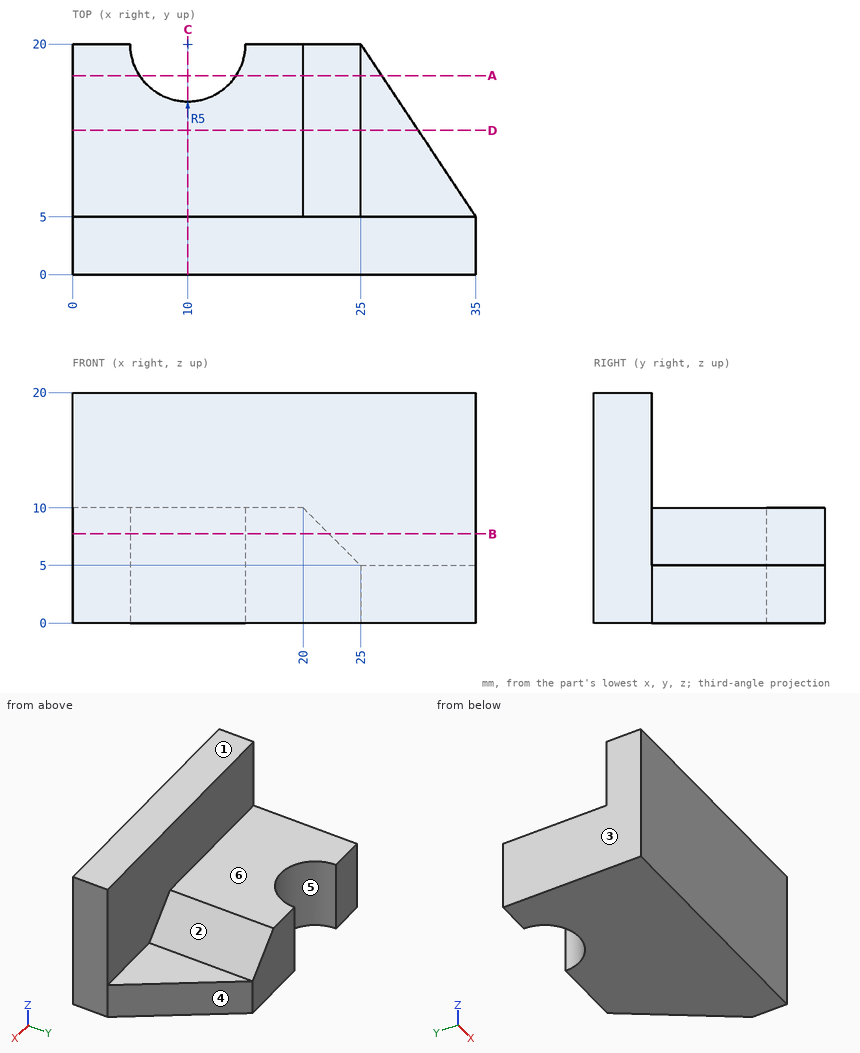
Could you check a few things on this drawing? It's one solid part, dimensions in mm from its lowest x, y, z. A direction names the side the tool comes from. Give positions to 0.01 mm unless a question says otherwise; leave off trailing zeros. Loops run counter-clockwise (first coordinate to the right, second up) from the corner with the lowest first, then second, coordinate; pieces in that order, holes last. Notation, with made-up numbers: (35.25, 48) -> (48.25, 48) arc R21 ccw to (48.25, 55) -> close; hole circle Ø5 at (-11.5, 47). An arc over 180 degrees is marked (long way). Use one line per item in the form item = value. Start each with the question number.
1) Please list where these lines run through material, in increasing order: line 1 along Y through (x, z) = (23, 11); line 2 along Z through (x, y) = (19, 18.5); line 3 along Y through (x, z) = (10, 6.75).
2) Imagine slicing it at C-C (x = 10). Please give me the cut outline in (y, z), then the cut area to 3 significant figures.
3) Imagine slicing it at D-D (y = 12.5). Please give me the cut outline in (x, z).
4) Imagine slicing it at A-A (y = 17.25). Please give me the cut outline in (x, z).
5) Which directions (+Z, -Z, +X, -X, +Y, -Y) give clear straight access to the entire face, cutting with the end or side of a thin tool? Please do the marked faces 1 and 2.
6) Imagine slicing it at B-B (z = 7.75). Please give me the cut outline in (x, y), then the cut area to 3 significant figures.
7) For P1, Ø5, axis at x = 29, y = 15.5, coming from the +Z side, with a flat end and sliding along its axis, tell me the tip position at first contact or that it passes through.
8) Thinking about a two-plate mould opening in X: for the marked faces 3, 4, 5 and 6, which applies, +X half, -X half, draft (parallel to the pull), parting line (faces both ways), or undercut?
Check values:
q1.line_1 = 0 to 5
q1.line_2 = 0 to 10
q1.line_3 = 0 to 15
q2.outline = (0, 0) -> (15, 0) -> (15, 10) -> (5, 10) -> (5, 20) -> (0, 20) -> close
q2.area = 200 mm^2
q3.outline = (0, 0) -> (30, 0) -> (30, 5) -> (25, 5) -> (20, 10) -> (0, 10) -> close
q4.outline = (0, 0) -> (5.82, 0) -> (5.82, 10) -> (0, 10) -> close; (14.18, 0) -> (26.83, 0) -> (26.83, 5) -> (25, 5) -> (20, 10) -> (14.18, 10) -> close
q5.face_1 = +Z, +X, -X, +Y, -Y
q5.face_2 = +Z, +X, +Y
q6.outline = (0, 0) -> (35, 0) -> (35, 5) -> (22.25, 5) -> (22.25, 20) -> (15, 20) arc R5 cw to (5, 20) -> (0, 20) -> close
q6.area = 469 mm^2
q7.P1 = 5
q8.face_3 = -X half
q8.face_4 = +X half
q8.face_5 = undercut
q8.face_6 = draft
